Check sheet for the drawn part. Datum: minimum x, y, z corner. Units: mm. Round coordinates to 2 decimals unless told otherwise and drop trailing zeros. Loops run counter-clockwise (first coordinate to the right, second up) from the corner with the lowest first, then second, coordinate; pieces in that order, holes last.
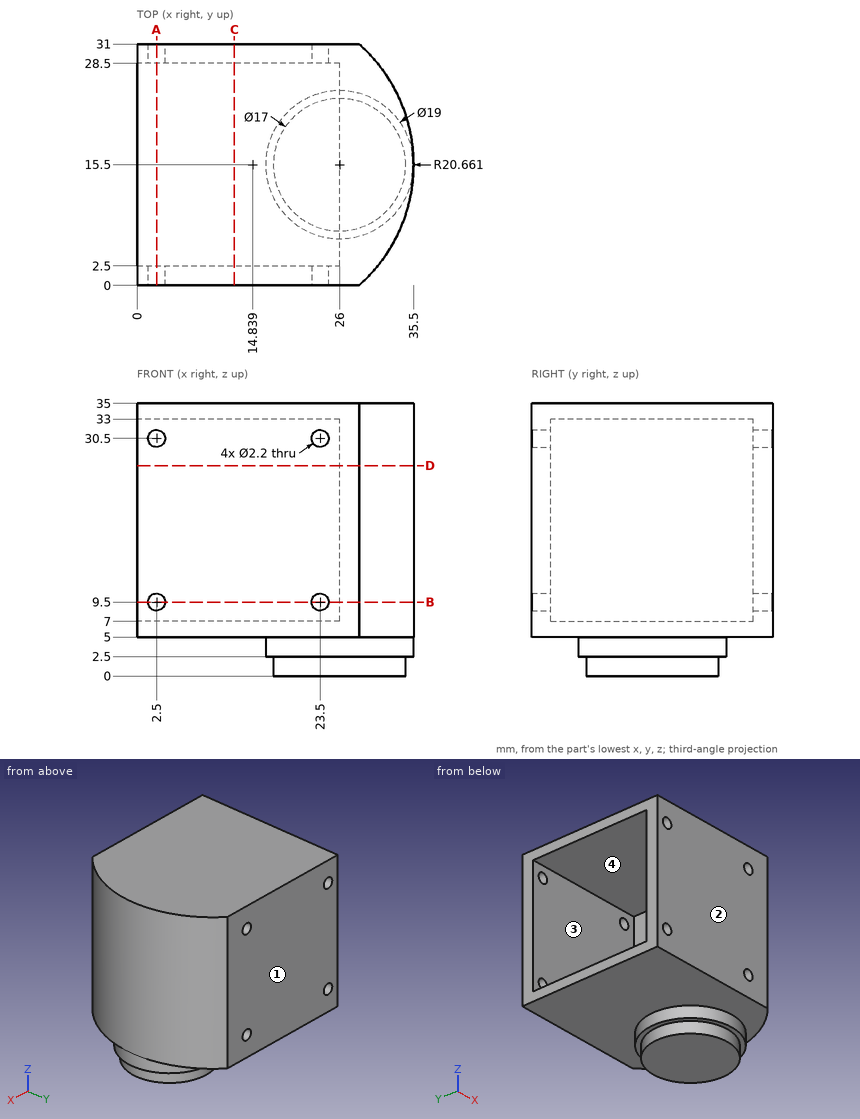
1) Sectioned sample at D-D, the plane z = 27. Record the cut outline in (x, y).
Report:
outline: (0, 0) - (28.5, 0) arc R20.66 ccw to (28.5, 31) - (0, 31) - (0, 28.5) - (26, 28.5) - (26, 2.5) - (0, 2.5) - close
2) Sectioned sample at B-B, the plane z = 9.5. Record the cut outline in (x, y).
Report:
outline: (0, 0) - (1.4, 0) - (1.4, 2.5) - (0, 2.5) - close; (0, 28.5) - (1.4, 28.5) - (1.4, 31) - (0, 31) - close; (3.6, 0) - (22.4, 0) - (22.4, 2.5) - (3.6, 2.5) - close; (3.6, 28.5) - (22.4, 28.5) - (22.4, 31) - (3.6, 31) - close; (24.6, 0) - (28.5, 0) arc R20.66 ccw to (28.5, 31) - (24.6, 31) - (24.6, 28.5) - (26, 28.5) - (26, 2.5) - (24.6, 2.5) - close
3) Gauge pin test, flat ends, axial feed: pin 1 (3.5 mm diameter, centred on x = 2.5, z = 9.5, fed in from +Y); pin 2 (10 mm diameter, centred on y = 25, z = 21, fed in from +X); pin 3 (8 mm diameter, centred on y = 19, z = 18, fed in from -X); pin 4 (3 mm diameter, centred on y = 26, z = 14.5, fed in from +X). Record the tip position at first contact, or that the pin passes through.
Report:
pin 1: stops at y = 31
pin 2: stops at x = 35
pin 3: stops at x = 26
pin 4: stops at x = 33.44
4) Sectioned sample at A-A, the plane x = 2.5. Record the cut outline in (y, z), then the cut area to 3 significant figures.
Report:
outline: (0, 5) - (31, 5) - (31, 8.4) - (28.5, 8.4) - (28.5, 7) - (2.5, 7) - (2.5, 8.4) - (0, 8.4) - close; (0, 10.6) - (2.5, 10.6) - (2.5, 29.4) - (0, 29.4) - close; (0, 31.6) - (2.5, 31.6) - (2.5, 33) - (28.5, 33) - (28.5, 31.6) - (31, 31.6) - (31, 35) - (0, 35) - close; (28.5, 10.6) - (31, 10.6) - (31, 29.4) - (28.5, 29.4) - close
area: 232 mm2
5) Mould release check, pull along Y, two halves, no side actions. Record for the marked faces 1, 2, 3 and 4: +Y half, -Y half, draft (parallel to the pull), parting line (faces both ways), or undercut.
Report:
face 1: +Y half
face 2: -Y half
face 3: undercut
face 4: undercut
6) Scan lines: line 1 along Z through (x, y) = (23.5, 30.3); line 2 along Y through (x, z) = (2, 27); line 3 along Z through (x, y) = (22, 27). Record each from-to range of solid material in increasing order.
Report:
line 1: z = 5 to 8.4, 10.6 to 29.4, 31.6 to 35
line 2: y = 0 to 2.5, 28.5 to 31
line 3: z = 5 to 7, 33 to 35
7) Sectioned sample at C-C, the plane x = 12.5. Record the cut outline in (y, z), then the cut area to 3 significant figures.
Report:
outline: (0, 5) - (31, 5) - (31, 35) - (0, 35) - close; hole (2.5, 7) - (28.5, 7) - (28.5, 33) - (2.5, 33) - close
area: 254 mm2
